from build123d import *

# Parameters (mm, degrees)
SKETCH_1_W             = 77.5
SKETCH_1_H             = 45
SKETCH_1_W_2           = 71.5
SKETCH_1_H_2           = 39
EXTRUDE_1_DEPTH        = 3
SKETCH_2_W             = 3
SKETCH_2_H             = 3
EXTRUDE_2_DEPTH        = 40
SKETCH_3_W             = 3
SKETCH_3_H             = 3
EXTRUDE_3_DEPTH        = 40
EXTRUDE_4_DEPTH        = 2
EXTRUDE_4_DEPTH_BACK   = 2
EXTRUDE_4_2_DEPTH      = 2
EXTRUDE_4_2_DEPTH_BACK = 2
SKETCH_5_W             = 65.5
SKETCH_5_H             = 6
EXTRUDE_5_DEPTH        = 3
SKETCH_6_W             = 65.5
SKETCH_6_H             = 6
EXTRUDE_6_DEPTH        = 3
SKETCH_7_R             = 1.5
CUT_EXTRUDE_1_DEPTH    = 5
CHAMFER_1_SIZE         = 0.5
CHAMFER_2_SIZE         = 0.5
CHAMFER_3_SIZE         = 2
CHAMFER_4_SIZE         = 2
EXTRUDE_7_DEPTH        = 6
MIRROR_2_COPY_1_DEPTH  = 6
SKETCH_9_W             = 2
SKETCH_9_H             = 45
CUT_EXTRUDE_2_DEPTH    = 10
FILLET_1_R             = 2


with BuildPart() as part:
    # Sketch 1 → Extrude 1 (new body)
    with BuildSketch(Plane.XY):
        Rectangle(SKETCH_1_W, SKETCH_1_H)
        Rectangle(SKETCH_1_W_2, SKETCH_1_H_2, mode=Mode.SUBTRACT)
    extrude(amount=EXTRUDE_1_DEPTH)

    # Sketch 2 → Extrude 2 (add)
    with BuildSketch(Plane.XY.offset(3)):
        with Locations((37.25, 21)):
            Rectangle(SKETCH_2_W, SKETCH_2_H)
        with Locations((-37.25, 21)):
            Rectangle(SKETCH_2_W, SKETCH_2_H)
        with Locations((-37.25, -21)):
            Rectangle(SKETCH_2_W, SKETCH_2_H)
        with Locations((37.25, -21)):
            Rectangle(SKETCH_2_W, SKETCH_2_H)
    extrude(amount=EXTRUDE_2_DEPTH)

    # Sketch 3 → Extrude 3 (add)
    with BuildSketch(Plane.XY.offset(3)):
        with Locations((-37.25, -18)):
            Rectangle(SKETCH_3_W, SKETCH_3_H)
        with Locations((-34.25, -21)):
            Rectangle(SKETCH_3_W, SKETCH_3_H)
        with Locations((34.25, -21)):
            Rectangle(SKETCH_3_W, SKETCH_3_H)
        with Locations((37.25, -18)):
            Rectangle(SKETCH_3_W, SKETCH_3_H)
        with Locations((37.25, 18)):
            Rectangle(SKETCH_3_W, SKETCH_3_H)
        with Locations((34.25, 21)):
            Rectangle(SKETCH_3_W, SKETCH_3_H)
        with Locations((-34.25, 21)):
            Rectangle(SKETCH_3_W, SKETCH_3_H)
        with Locations((-37.25, 18)):
            Rectangle(SKETCH_3_W, SKETCH_3_H)
    extrude(amount=EXTRUDE_3_DEPTH)

    # Sketch 5 → Extrude 5 (add)
    with BuildSketch(Plane(origin=(0, 22.5, 0), x_dir=(1, 0, 0), z_dir=(0, 1, 0))):
        with Locations((0, -6)):
            Rectangle(SKETCH_5_W, SKETCH_5_H)
    extrude(amount=-EXTRUDE_5_DEPTH)


with BuildPart() as body_2:
    # Sketch 4 → Extrude 4 (new, two sides: drawn at the far end of the back side and taken through both)
    with BuildSketch(Plane.XY.offset(43).offset(-EXTRUDE_4_DEPTH_BACK)):
        Polygon((38.75, 22.5), (53.75, 22.5), (53.75, -22.5), (38.75, -22.5), (38.75, -16.5), (39.5, -16.5), (39.5, 16.5), (38.75, 16.5), align=None)
    extrude(amount=EXTRUDE_4_DEPTH + EXTRUDE_4_DEPTH_BACK)


with BuildPart() as body_3:
    # Sketch 4 → Extrude 4 2 (new, two sides: drawn at the far end of the back side and taken through both)
    with BuildSketch(Plane.XY.offset(43).offset(-EXTRUDE_4_2_DEPTH_BACK)):
        Polygon((-38.75, -16.5), (-38.75, -22.5), (-53.75, -22.5), (-53.75, 22.5), (-38.75, 22.5), (-38.75, 16.5), (-39.5, 16.5), (-39.5, -16.5), align=None)
    extrude(amount=EXTRUDE_4_2_DEPTH + EXTRUDE_4_2_DEPTH_BACK)


with BuildPart() as body_4:
    # Sketch 6 → Extrude 6 (new body)
    with BuildSketch(Plane.XZ.offset(22.5)):
        with Locations((0, 6)):
            Rectangle(SKETCH_6_W, SKETCH_6_H)
    extrude(amount=-EXTRUDE_6_DEPTH)


with BuildPart() as cut_extrude_1_tool:
    # Sketch 7 → Cut-Extrude 1 (new body)
    with BuildSketch(Plane.XY.offset(45)):
        with Locations((-46, 0)):
            Circle(SKETCH_7_R)
        with Locations((46, 0)):
            Circle(SKETCH_7_R)
    extrude(amount=-CUT_EXTRUDE_1_DEPTH)


with BuildPart() as body_2_1:
    add(body_2.part)

    # Cut-Extrude 1: cut by cut_extrude_1_tool
    add(cut_extrude_1_tool.part, mode=Mode.SUBTRACT)

    # Chamfer 2
    chamfer_2_edges = [body_2_1.edges().sort_by_distance(p)[0] for p in [
        (44.5, 0, 45),
    ]]
    chamfer(chamfer_2_edges, length=CHAMFER_2_SIZE)

    # Chamfer 3
    chamfer_3_edges = [body_2_1.edges().sort_by_distance(p)[0] for p in [
        (53.75, 22.5, 43),
        (53.75, -22.5, 43),
    ]]
    chamfer(chamfer_3_edges, length=CHAMFER_3_SIZE)


with BuildPart() as body_3_1:
    add(body_3.part)

    # Cut-Extrude 1: cut by cut_extrude_1_tool
    add(cut_extrude_1_tool.part, mode=Mode.SUBTRACT)

    # Chamfer 1
    chamfer_1_edges = [body_3_1.edges().sort_by_distance(p)[0] for p in [
        (-47.5, 0, 45),
    ]]
    chamfer(chamfer_1_edges, length=CHAMFER_1_SIZE)


with BuildPart() as part_1:
    add(part.part)

    # Combine 1: union body 3
    add(body_3_1.part)


with BuildPart() as body_4_1:
    add(body_4.part)

    # Combine 2: union part
    add(part_1.part)


with BuildPart() as body_2_2:
    add(body_2_1.part)

    # Combine 3: union body 4
    add(body_4_1.part)

    # Chamfer 4
    chamfer_4_edges = [body_2_2.edges().sort_by_distance(p)[0] for p in [
        (-53.75, 22.5, 43),
        (-53.75, -22.5, 43),
    ]]
    chamfer(chamfer_4_edges, length=CHAMFER_4_SIZE)

    # Sketch 8 → Extrude 7 (add)
    with BuildSketch(Plane(origin=(0, 22.5, 0), x_dir=(1, 0, 0), z_dir=(0, 1, 0))):
        Polygon((48.75, -41), (38.75, -26), (38.75, -41), align=None)
    extrude_7 = extrude(amount=-EXTRUDE_7_DEPTH)

    # Mirror 1: Extrude 7 across plane
    add(extrude_7.mirror(Plane(origin=(0, 0, 0), x_dir=(0, 0, 1), z_dir=(1, 0, 0))))

    # Mirror 2: Extrude 7 across plane
    add(extrude_7.mirror(Plane.ZX))

    # Mirror 2 copy 1 sketch → Mirror 2 copy 1 (add)
    with BuildSketch(Plane(origin=(0, -22.5, 0), x_dir=(-1, 0, 0), z_dir=(0, -1, 0))):
        Polygon((48.75, -41), (38.75, -26), (38.75, -41), align=None)
    extrude(amount=-MIRROR_2_COPY_1_DEPTH)

    # Sketch 9 → Cut-Extrude 2 (cut)
    with BuildSketch(Plane(origin=(0, 0, 41), x_dir=(-1, 0, 0), z_dir=(0, 0, -1))):
        with Locations((52.75, 0)):
            Rectangle(SKETCH_9_W, SKETCH_9_H)
        with Locations((-52.75, 0)):
            Rectangle(SKETCH_9_W, SKETCH_9_H)
    extrude(amount=-CUT_EXTRUDE_2_DEPTH, mode=Mode.SUBTRACT)

    # Fillet 1
    fillet_1_edges = [body_2_2.edges().sort_by_distance(p)[0] for p in [
        (-51.75, -22.5, 43),
        (-51.75, 22.5, 43),
        (51.75, -22.5, 43),
        (51.75, 22.5, 43),
    ]]
    fillet(fillet_1_edges, radius=FILLET_1_R)


solid = body_2_2.part
Work out the finished part from the listing and answer in its coordinate system (mm). A direction names the side the tool comes from. Coordinates: 2 decimals unless noted, no trailing zeros. Loops run counter-clockwise (first coordinate to the right, second up) from the corner with the lowest first, then second, coordinate; pieces in that order, holes last. Notation, with made-up numbers: M -34.5,53.5 L -1.5,53.5 A24 cw -1.5,85.5 Z; hole C -34,-33.5 d2. An arc over 180 degrees is marked long. Answer in a Markdown table with one row per item. Add a question column.
1. Consider L1, parallel to Y at x = -46, z = 42; L2, parallel to X at y = 20, z = 25; L3, parallel to Y at x = 33, z = 30. Determine where each line is inside the solid, lowest interval first.
2. A tool of negligible diameter and unlimited length cuts with its end or side. For faces 1 (the flat face through (32.75, 21, 26)), 2 (the flat face through (37, 0, 3)), 3 (the flat face through (-39.5, 0, 43)), 4 (the flat face through (38.75, -0.1, 0.4)), from which of +Z, -Z, +X, -X, +Y, -Y can it reach the whole face along a straight path? Write none if from no direction.
3. Flat-ended cylindrical pins translate along their axes: P1, Ø14.5, axis at x = 43.5, z = 26.5, coming from the -Y side; P2, Ø1.5, axis at y = -21, z = 29.5, coming from the +X side; P3, Ø19.5, axis at y = 8.5, z = 24, coming from the -X side; P4, Ø12, axis at x = -26, z = 37.5, coming from the +Y side. Find the tip coordinate at first contact, or state that the pin passes through.
4. Find section D-D, the plane z = 17.5. Write down the section's boundary in (x, y), then the cut area to 3 significant figures.
5. Find section A-A, the plane y = 0. Write down the section's boundary in (x, z), then the cut area to 3 significant figures.
6. Find section C-C, the plane x = 12. Write down the section's boundary in (y, z).
7. The mould has two halves that part along Y. Classify faces 5 (the flat face through (0, -22.5, 6)), 6 (the flat face through (-35.75, -3, 2)), 7 (the flat face through (-51.75, 0, 43)), 8 (the flat face through (39.5, 0, 43)): pulls with the +Y half, pulls with the -Y half, needs draft (parallel to the pull), parting line crosses it, or undercut.
8. Find section B-B, the plane y = 18. Write down the section's boundary in (x, z), then the cut area to 3 significant figures.
Reported:
| question | item | result |
|---|---|---|
| 1 | L1 | y = -22.5 to -1.5, 1.5 to 22.5 |
| 1 | L2 | x = -38.75 to -32.75, 32.75 to 38.75 |
| 1 | L3 | y = -22.5 to -19.5, 19.5 to 22.5 |
| 2 | face 1 | +Z, +Y, -Y |
| 2 | face 2 | +Z, +X, -X |
| 2 | face 3 | +Z, -Z |
| 2 | face 4 | -Z, +X, +Y, -Y |
| 3 | P1 | stops at y = -22.5 |
| 3 | P2 | stops at x = 41.58 |
| 3 | P3 | stops at x = -41.13 |
| 3 | P4 | passes through |
| 4 | outline | M -38.75,-22.5 L -32.75,-22.5 L -32.75,-19.5 L -35.75,-19.5 L -35.75,-16.5 L -38.75,-16.5 Z; M -38.75,16.5 L -35.75,16.5 L -35.75,19.5 L -32.75,19.5 L -32.75,22.5 L -38.75,22.5 Z; M 32.75,-22.5 L 38.75,-22.5 L 38.75,-16.5 L 35.75,-16.5 L 35.75,-19.5 L 32.75,-19.5 Z; M 32.75,19.5 L 35.75,19.5 L 35.75,16.5 L 38.75,16.5 L 38.75,22.5 L 32.75,22.5 Z |
| 4 | area | 108 mm^2 |
| 5 | outline | M -51.75,41 L -47.5,41 L -47.5,44.5 L -48,45 L -51.75,45 Z; M -44.5,41 L -39.5,41 L -39.5,45 L -44,45 L -44.5,44.5 Z; M -38.75,0 L -35.75,0 L -35.75,3 L -38.75,3 Z; M 35.75,0 L 38.75,0 L 38.75,3 L 35.75,3 Z; M 39.5,41 L 44.5,41 L 44.5,44.5 L 44,45 L 39.5,45 Z; M 47.5,41 L 51.75,41 L 51.75,45 L 48,45 L 47.5,44.5 Z |
| 5 | area | 91.5 mm^2 |
| 6 | outline | M -22.5,0 L -19.5,0 L -19.5,9 L -22.5,9 Z; M 19.5,0 L 22.5,0 L 22.5,9 L 19.5,9 Z |
| 7 | face 5 | pulls with the -Y half |
| 7 | face 6 | undercut |
| 7 | face 7 | needs draft |
| 7 | face 8 | undercut |
| 8 | outline | M -51.75,41 L -48.75,41 L -38.75,26 L -38.75,0 L -35.75,0 L -35.75,43 L -38.75,43 L -38.75,45 L -51.75,45 Z; M 35.75,0 L 38.75,0 L 38.75,26 L 48.75,41 L 51.75,41 L 51.75,45 L 38.75,45 L 38.75,43 L 35.75,43 Z |
| 8 | area | 512 mm^2 |
